Source: CAD feature listing. Evaluate the final solid. Frame: model axes, mm. Round coordinates to 2 decimals unless told otherwise and drop trailing zeros. Order: outer loops, then holes, each group sorted by start corner. A loop starts at its lowest first (then second) coordinate and runs counter-clockwise, first axis right, second up. Notation, with made-up numbers: (-36, 25.5) -> (-26, 25.5) arc R30 ccw to (-26, 53.5) -> close; hole circle Ø11 at (-29.75, 85). An arc over 180 degrees is marked (long way). Write item = value, one per line. Start each with the question number.
(1) Cut plane B-B on y = -1.05. Return the cut outline in (x, z) (1 decimal), then the cut area to 3 significant figures.
(2) Ray query, line 1 (X direction, y = -1.2, z = 0.25); line 2 (X direction, y = -0.55, z = -1.25); line 3 (Z direction, x = 58, y = -0.8). Return the intervals inside material, ascending.
(3) Cut plane A-A on z = 0. Return the cut outline in (x, y), then the cut area to 3 significant figures.
(4) Contact query for a flat-ended pin moving along its axis: pin 1 Ø5 at (x, z) = (58.674, 0) entering from +Y. Output: stop coordinate, or through.
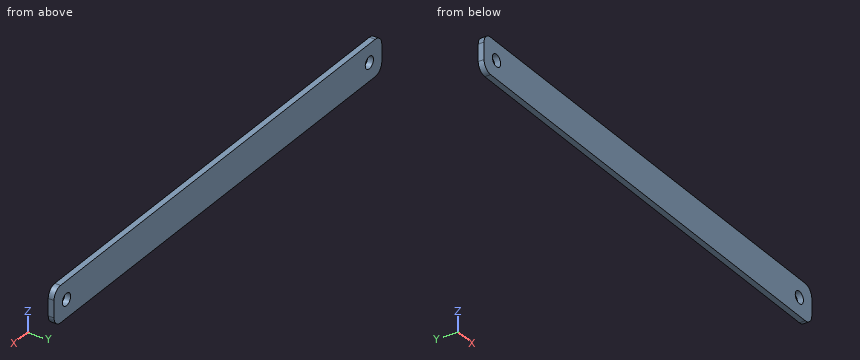
from build123d import *

# Parameters (mm, degrees)
F0_W     = 127
F0_H     = 9.525
F1_DEPTH = 1.524
F2_R     = 2.54
F4_D     = 3.175
F4_DEPTH = 19.05


with BuildPart() as f1:
    # F0 (on Front) → F1 (new body)
    with BuildSketch(Plane.XZ):
        Rectangle(F0_W, F0_H)
    extrude(amount=F1_DEPTH)

    # F2
    f2_edges = [f1.edges().sort_by_distance(p)[0] for p in [
        (-63.5, -0.762, 4.7625),
        (-63.5, -0.762, -4.7625),
        (63.5, -0.762, -4.7625),
        (63.5, -0.762, 4.7625),
    ]]
    fillet(f2_edges, radius=F2_R)

    # F4
    with Locations(Plane.XZ.offset(1.524)):
        with Locations((-58.674, 0), (58.674, 0)):
            Hole(F4_D / 2, depth=F4_DEPTH)


solid = f1.part
Evaluation:
q1.outline = (-63.5, -2.2) arc R2.5 ccw to (-61, -4.8) -> (61, -4.8) arc R2.5 ccw to (63.5, -2.2) -> (63.5, 2.2) arc R2.5 ccw to (61, 4.8) -> (-61, 4.8) arc R2.5 ccw to (-63.5, 2.2) -> close; hole circle Ø3.2 at (-58.7, 0); hole circle Ø3.2 at (58.7, 0)
q1.area = 1,190 mm^2
q2.line_1 = -63.5 to -60.24, -57.11 to 57.11, 60.24 to 63.5
q2.line_2 = -63.5 to -59.65, -57.7 to 57.7, 59.65 to 63.5
q2.line_3 = -4.76 to -1.44, 1.44 to 4.76
q3.outline = (-63.5, -1.52) -> (-60.26, -1.52) -> (-60.26, 0) -> (-63.5, 0) -> close; (-57.09, -1.52) -> (57.09, -1.52) -> (57.09, 0) -> (-57.09, 0) -> close; (60.26, -1.52) -> (63.5, -1.52) -> (63.5, 0) -> (60.26, 0) -> close
q3.area = 184 mm^2
q4.pin_1 = 0
